Can you work these out from the model? Positions are in its coordinate system, mm. Give positions to 0.01 mm unless a question says otherwise; leave off trailing zeros. Loops run counter-clockwise (first coordinate to the right, second up) from the corner with the lowest first, then second, coordinate; pieces in that order, holes last. Notation, with made-up numbers: M 32.5,0 L 87.5,0 A22 cw 87.5,37 Z; hole C 83.25,73 d7. An arc over 180 degrees is marked long. Use CSV: the item, a comma, the result in double quotes.
from build123d import *

# Parameters (mm, degrees)
SKETCH1_W                = 139.7
SKETCH1_H                = 12.7
BOSS_EXTRUDE1_DEPTH      = 6.35
H_0_266_DIAMETER_HOLE1_D = 6.7564
FILLET1_R                = 2.54


with BuildPart() as part:
    # Sketch1 → Boss-Extrude1 (new body)
    with BuildSketch(Plane.XY):
        Rectangle(SKETCH1_W, SKETCH1_H)
    extrude(amount=BOSS_EXTRUDE1_DEPTH)

    # H (0.266) Diameter Hole1 (through all)
    with Locations(Plane.XY.offset(6.35)):
        with Locations((-64.77, 0), (-52.07, 0), (52.07, 0), (64.77, 0)):
            Hole(H_0_266_DIAMETER_HOLE1_D / 2)

    # Fillet1
    fillet1_edges = [part.edges().sort_by_distance(p)[0] for p in [
        (69.85, -6.35, 3.175),
        (-69.85, -6.35, 3.175),
        (-69.85, 6.35, 3.175),
        (69.85, 6.35, 3.175),
    ]]
    fillet(fillet1_edges, radius=FILLET1_R)


solid = part.part
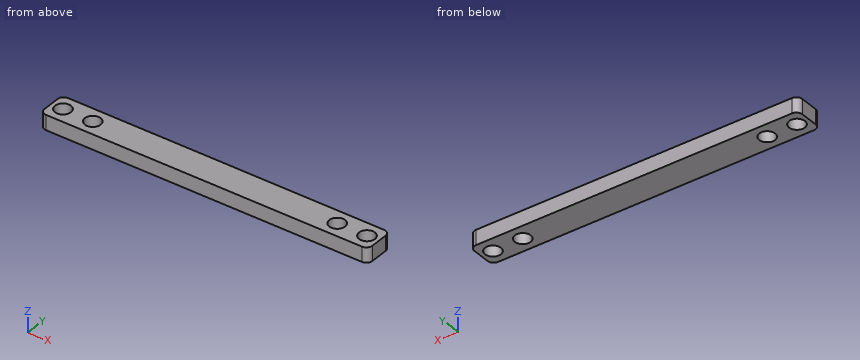
Q1. I want a section at C-C, the plane z = 2.25. Please give me the cut outline in (x, y).
Model answer:
outline,"M -69.85,-3.81 A2.54 ccw -67.31,-6.35 L 67.31,-6.35 A2.54 ccw 69.85,-3.81 L 69.85,3.81 A2.54 ccw 67.31,6.35 L -67.31,6.35 A2.54 ccw -69.85,3.81 Z; hole C -64.77,0 d6.76; hole C -52.07,0 d6.76; hole C 52.07,0 d6.76; hole C 64.77,0 d6.76"
Q2. I'm going to push a flat-ended pin straight in: P1, Ø5.5, axis at x = 64.77, y = 0, coming from the -Z side. Where does the tip first touch, or does it pass through?
Model answer:
P1,"through"
Q3. I want a section at B-B, the plane y = 0. Please give me the cut outline in (x, z), then the cut area to 3 significant figures.
Model answer:
outline,"M -69.85,0 L -68.15,0 L -68.15,6.35 L -69.85,6.35 Z; M -61.39,0 L -55.45,0 L -55.45,6.35 L -61.39,6.35 Z; M -48.69,0 L 48.69,0 L 48.69,6.35 L -48.69,6.35 Z; M 55.45,0 L 61.39,0 L 61.39,6.35 L 55.45,6.35 Z; M 68.15,0 L 69.85,0 L 69.85,6.35 L 68.15,6.35 Z"
area,"715 mm2"
Q4. I want a section at A-A, the plane x = 52.07. Please give me the cut outline in (y, z).
Model answer:
outline,"M -6.35,0 L -3.38,0 L -3.38,6.35 L -6.35,6.35 Z; M 3.38,0 L 6.35,0 L 6.35,6.35 L 3.38,6.35 Z"
Q5. Please list where these lines run through material, in increasing order: L1, parallel to Y at x = -52.07, z = 3.75; L2, parallel to X at y = -2, z = 6.25; L3, parallel to X at y = 4, z = 6.25. Write a range as from..to.
Model answer:
L1,"-6.35..-3.38, 3.38..6.35"
L2,"-69.85..-67.49, -62.05..-54.79, -49.35..49.35, 54.79..62.05, 67.49..69.85"
L3,"-69.84..69.84"
